Part model, mm, in its own coordinate system. A direction names the side the tool comes from. Coordinates: 2 decimals unless noted, no trailing zeros. Loops run counter-clockwise (first coordinate to the right, second up) from the corner with the lowest first, then second, coordinate; pieces in that order, holes last. Notation, with made-up numbers: M 37,30.25 L 84,30.25 A31 ccw 84,59.25 Z; hole C 55,34.5 d4. An arc over 180 degrees is marked long. Answer as a JSON object with one key per item and string values. Group by question number.
1. Drill centre lines: L1, parallel to X at y = 21.9, z = 20; L2, parallel to Z at x = -1, y = 21; L3, parallel to Y at x = 0.5, z = 22.5. Where is each one in solid material? Low to high.
2. Saw through at C-C on z = 17. Write the cut outline in (x, y), then the cut area to 3 significant figures.
3. Mould opens along X. For faces 1 (the face through (0, -6, 12.5)), 2 (the face through (8, 19, -19)), 3 (the face through (1.526, -0.481, -83.028)) say: released by +X, released by -X, zero draft, split by the parting line, or undercut.
4. Saw through at B-B on x = -3.75. Write the cut outline in (y, z), then the cut area to 3 significant figures.
5. Saw through at A-A on z = -65. Write the cut outline in (x, y).
6. 3-axis set-ups, long thin cutter, end or side, ignore diameter. For faces 4 (the face through (0, 6, 26)), 5 (the face through (0, -5, 28)), 6 (the face through (-1.27, -0.97, 28.03)), 7 (the face through (0.11, 10.33, 14.74)): which of +Z, -Z, +X, -X, +Y, -Y reach the whole face in a straight line?
7. Drop flat-ended pins along their axis: pin 1 Ø1.2 at (x, z) = (-0.5, 29) entering from -Y; pin 2 Ø1.3 at (x, y) = (-1, -6) entering from -Z; pin 3 Ø1 at (x, z) = (5.5, -54) entering from -Y; pin 4 Ø1.9 at (x, z) = (0, -65) entering from +Y. Give the stop position or say it passes through.
8. Saw through at D-D on z = -44. Write the cut outline in (x, y).
from build123d import *

# Parameters (mm, degrees)
BOSS_EXTRUDE1_DEPTH = 8
CHAMFER1_SIZE       = 2
CHAMFER2_SIZE       = 2
CUT_EXTRUDE1_REACH  = 119.55
SKETCH2_R           = 1.6
CUT_EXTRUDE2_REACH  = 119.55
SKETCH3_R           = 1.6
CUT_EXTRUDE3_REACH  = 93.531
SKETCH4_R           = 1.6


with BuildPart() as part:
    # Sketch1 → Boss-Extrude1 (new, symmetric)
    with BuildSketch(Plane(origin=(0, 0, 0), x_dir=(0, 0, -1), z_dir=(1, 0, 0))):
        with BuildLine():
            Line((-12.5, -3.570714214), (-12.5, -10))
            Line((-12.5, -10), (-18, -10))
            Line((-18, -10), (-18, 0))
            ThreePointArc((-18, 0), (-14.647202482, 10.462287487), (-5.837837838, 17.027027027))
            ThreePointArc((-5.837837838, 17.027027027), (-5.506803038, 17.582199494), (-6, 18))
            Line((-6, 18), (-26, 18))
            Line((-26, 18), (-26, -5))
            Line((-26, -5), (-30, -5))
            Line((-30, -5), (-30, 18))
            Line((-30, 18), (-30, 23))
            Line((-30, 23), (85, 23))
            Line((85, 23), (85, 18))
            Line((85, 18), (85, -5))
            Line((85, -5), (81, -5))
            Line((81, -5), (81, 18))
            Line((81, 18), (6, 18))
            ThreePointArc((6, 18), (5.506803038, 17.582199494), (5.837837838, 17.027027027))
            ThreePointArc((5.837837838, 17.027027027), (14.647202482, 10.462287487), (18, 0))
            Line((18, 0), (18, -10))
            Line((18, -10), (12.5, -10))
            Line((12.5, -10), (12.5, -3.570714214))
            ThreePointArc((12.5, -3.570714214), (0, 13), (-12.5, -3.570714214))
        make_face()
    extrude(amount=BOSS_EXTRUDE1_DEPTH, both=True)

    # Chamfer1
    chamfer1_edges = [part.edges().sort_by_distance(p)[0] for p in [
        (0, 18, 26),
        (0, 18, -81),
    ]]
    chamfer(chamfer1_edges, length=CHAMFER1_SIZE)

    # Chamfer2
    chamfer2_edges = [part.edges().sort_by_distance(p)[0] for p in [
        (0, -10, -12.5),
        (0, -10, 12.5),
        (0, 23, 30),
        (0, 23, -85),
    ]]
    chamfer(chamfer2_edges, length=CHAMFER2_SIZE)

    # Sketch2 → Cut-Extrude1 (cut, up to next)
    with BuildSketch(Plane.XY.offset(30), mode=Mode.PRIVATE) as cut_extrude1_sk1:
        Circle(SKETCH2_R)
    cut_extrude1_tool1 = extrude(cut_extrude1_sk1.sketch, amount=-CUT_EXTRUDE1_REACH, mode=Mode.PRIVATE) & part.part
    add(cut_extrude1_tool1.solids().sort_by_distance((0, 0, 30))[0], mode=Mode.SUBTRACT)

    # Sketch3 → Cut-Extrude2 (cut, up to next)
    with BuildSketch(Plane(origin=(0, 0, -85), x_dir=(-1, 0, 0), z_dir=(0, 0, -1)), mode=Mode.PRIVATE) as cut_extrude2_sk1:
        with Locations(Location((0, 0, 0), (0, 0, 180))):
            Circle(SKETCH3_R)
    cut_extrude2_tool1 = extrude(cut_extrude2_sk1.sketch, amount=-CUT_EXTRUDE2_REACH, mode=Mode.PRIVATE) & part.part
    add(cut_extrude2_tool1.solids().sort_by_distance((0, 0, -85))[0], mode=Mode.SUBTRACT)

    # Sketch4 → Cut-Extrude3 (cut, up to next)
    with BuildSketch(Plane(origin=(0, 23, 0), x_dir=(1, 0, 0), z_dir=(0, 1, 0)), mode=Mode.PRIVATE) as cut_extrude3_sk1:
        with Locations(Location((0, 65, 0), (0, 0, 270))):
            Circle(SKETCH4_R)
    cut_extrude3_tool1 = extrude(cut_extrude3_sk1.sketch, amount=-CUT_EXTRUDE3_REACH, mode=Mode.PRIVATE) & part.part
    # Sketch4 → Cut-Extrude3 (cut, up to next)
    with BuildSketch(Plane(origin=(0, 23, 0), x_dir=(1, 0, 0), z_dir=(0, 1, 0)), mode=Mode.PRIVATE) as cut_extrude3_sk2:
        with Locations(Location((0, 25, 0), (0, 0, 270))):
            Circle(SKETCH4_R)
    cut_extrude3_tool2 = extrude(cut_extrude3_sk2.sketch, amount=-CUT_EXTRUDE3_REACH, mode=Mode.PRIVATE) & part.part
    # Sketch4 → Cut-Extrude3 (cut, up to next)
    with BuildSketch(Plane(origin=(0, 23, 0), x_dir=(1, 0, 0), z_dir=(0, 1, 0)), mode=Mode.PRIVATE) as cut_extrude3_sk3:
        with Locations(Location((0, -20, 0), (0, 0, 270))):
            Circle(SKETCH4_R)
    cut_extrude3_tool3 = extrude(cut_extrude3_sk3.sketch, amount=-CUT_EXTRUDE3_REACH, mode=Mode.PRIVATE) & part.part
    add(cut_extrude3_tool1.solids().sort_by_distance((0, 23, -65))[0], mode=Mode.SUBTRACT)
    add(cut_extrude3_tool2.solids().sort_by_distance((0, 23, -25))[0], mode=Mode.SUBTRACT)
    add(cut_extrude3_tool3.solids().sort_by_distance((0, 23, 20))[0], mode=Mode.SUBTRACT)


solid = part.part
Outcome:
{
 "1": {"L1": "x = -8 to -1.6, 1.6 to 8", "L2": "z = -85 to -66.25, -63.75 to -26.25, -23.75 to 18.75, 21.25 to 30", "L3": "y = 18 to 23"},
 "2": {"outline": "M -8,-10 L 8,-10 L 8,5.92 L -8,5.92 Z; M -8,18 L 8,18 L 8,23 L -8,23 Z", "area": "335 mm²"},
 "3": {"face 1": "zero draft", "face 2": "released by +X", "face 3": "undercut"},
 "4": {"outline": "M -10,-18 L 0,-18 A18 ccw 17.03,-5.84 A0.5 cw 18,-6 L 18,-79 L 16,-81 L -5,-81 L -5,-85 L 21,-85 L 23,-83 L 23,28 L 21,30 L -5,30 L -5,26 L 16,26 L 18,24 L 18,6 A0.5 cw 17.03,5.84 A18 ccw 0,18 L -10,18 L -10,14.5 L -8,12.5 L -3.57,12.5 A13 cw long -3.57,-12.5 L -8,-12.5 L -10,-14.5 Z", "area": "1,110 mm²"},
 "5": {"outline": "M -8,18 L -1.6,18 L -1.6,23 L -8,23 Z; M 1.6,18 L 8,18 L 8,23 L 1.6,23 Z"},
 "6": {"face 4": "+X, -X, -Y", "face 5": "+Z, +X, -X, -Y", "face 6": "+Z", "face 7": "+X, -X"},
 "7": {"pin 1": "stops at y = -5", "pin 2": "stops at z = -18", "pin 3": "stops at y = 18", "pin 4": "passes through"},
 "8": {"outline": "M -8,18 L 8,18 L 8,23 L -8,23 Z"}
}
